```python
from build123d import *

# Parameters (mm, degrees)
SKETCH1_R           = 3.3655
SKETCH1_R_2         = 2.2352
BOSS_EXTRUDE1_DEPTH = 2.54
SKETCH2_R           = 0.6604
SKETCH2_R_2         = 2.31775
SKETCH2_R_3         = 3.3655
SKETCH2_R_4         = 2.2352
SKETCH2_R_5         = 1.143
BOSS_EXTRUDE2_DEPTH = 1.7272
FILLET1_R           = 12.7
SKETCH3_R           = 2.06375
SKETCH3_R_2         = 1.143
CUT_EXTRUDE1_DEPTH  = 1.27
SKETCH8_R           = 0.98
CUT_EXTRUDE4_DEPTH  = 20.062316393


with BuildPart() as part:
    # Sketch1 → Boss-Extrude1 (new body)
    with BuildSketch(Plane(origin=(0, 0, 0), x_dir=(1, 0, 0), z_dir=(0, 1, 0))):
        with Locations(Location((0, 0, 0), (0, 0, 270))):
            Circle(SKETCH1_R)
        with Locations(Location((0, 0, 0), (0, 0, 270))):
            Circle(SKETCH1_R_2, mode=Mode.SUBTRACT)
    extrude(amount=BOSS_EXTRUDE1_DEPTH)

    # Sketch2 → Boss-Extrude2 (add)
    with BuildSketch(Plane(origin=(0, 2.54, 0), x_dir=(1, 0, 0), z_dir=(0, 1, 0))):
        with BuildLine():
            ThreePointArc((-0.713521748, -3.755518873), (-3.8227, 0), (-0.713521748, 3.755518873))
            Line((-0.713521748, 3.755518873), (-16.092265178, 2.307544345))
            ThreePointArc((-16.092265178, 2.307544345), (-14.314807913, 1.713991165), (-13.55725, 0))
            ThreePointArc((-13.55725, 0), (-14.314807913, -1.713991165), (-16.092265178, -2.307544345))
            Line((-16.092265178, -2.307544345), (-0.713521748, -3.755518873))
        make_face()
        with Locations(Location((-12.8778, 0, 0), (0, 0, 270))):
            Circle(SKETCH2_R, mode=Mode.SUBTRACT)
        with Locations(Location((-9.8806, 0, 0), (0, 0, 270))):
            Circle(SKETCH2_R, mode=Mode.SUBTRACT)
        with Locations(Location((-7.1628, 0, 0), (0, 0, 270))):
            Circle(SKETCH2_R, mode=Mode.SUBTRACT)
        with Locations((-15.875, 0)):
            Circle(SKETCH2_R_2)
        with Locations(Location((-15.875, 0, 0), (0, 0, 270))):
            Circle(SKETCH2_R, mode=Mode.SUBTRACT)
        with BuildLine():
            Line((16.092265178, 2.307544345), (0.713521748, 3.755518873))
            ThreePointArc((0.713521748, 3.755518873), (2.944538578, 2.437771083), (3.8227, 0))
            ThreePointArc((3.8227, 0), (2.944538578, -2.437771083), (0.713521748, -3.755518873))
            Line((0.713521748, -3.755518873), (16.092265178, -2.307544345))
            ThreePointArc((16.092265178, -2.307544345), (13.55725, 0), (16.092265178, 2.307544345))
        make_face()
        with Locations(Location((7.1628, 0, 0), (0, 0, 270))):
            Circle(SKETCH2_R, mode=Mode.SUBTRACT)
        with Locations(Location((9.8806, 0, 0), (0, 0, 270))):
            Circle(SKETCH2_R, mode=Mode.SUBTRACT)
        with Locations(Location((12.8778, 0, 0), (0, 0, 270))):
            Circle(SKETCH2_R, mode=Mode.SUBTRACT)
        with Locations((15.875, 0)):
            Circle(SKETCH2_R_2)
        with Locations(Location((15.875, 0, 0), (0, 0, 270))):
            Circle(SKETCH2_R, mode=Mode.SUBTRACT)
        with BuildLine():
            Line((0.713521748, 3.755518873), (0, 3.8227))
            Line((0, 3.8227), (-0.713521748, 3.755518873))
            ThreePointArc((-0.713521748, 3.755518873), (-3.8227, 0), (-0.713521748, -3.755518873))
            Line((-0.713521748, -3.755518873), (0, -3.8227))
            Line((0, -3.8227), (0.713521748, -3.755518873))
            ThreePointArc((0.713521748, -3.755518873), (2.944538578, -2.437771083), (3.8227, 0))
            ThreePointArc((3.8227, 0), (2.944538578, 2.437771083), (0.713521748, 3.755518873))
        make_face()
        with Locations(Location((0, 0, 0), (0, 0, 270))):
            Circle(SKETCH2_R_3, mode=Mode.SUBTRACT)
        with Locations(Location((0, 0, 0), (0, 0, 270))):
            Circle(SKETCH2_R_3)
        with Locations(Location((0, 0, 0), (0, 0, 270))):
            Circle(SKETCH2_R_4, mode=Mode.SUBTRACT)
        with Locations(Location((0, 0, 0), (0, 0, 270))):
            Circle(SKETCH2_R_4)
        with Locations(Location((0, 0, 0), (0, 0, 270))):
            Circle(SKETCH2_R_5, mode=Mode.SUBTRACT)
    extrude(amount=BOSS_EXTRUDE2_DEPTH)

    # Fillet1
    fillet1_edges = [part.edges().sort_by_distance(p)[0] for p in [
        (0, 3.4036, -3.8227),
        (0, 3.4036, 3.8227),
    ]]
    fillet(fillet1_edges, radius=FILLET1_R)

    # Sketch3 → Cut-Extrude1 (cut)
    with BuildSketch(Plane(origin=(0, 4.2672, 0), x_dir=(1, 0, 0), z_dir=(0, 1, 0))):
        with Locations(Location((0, 0, 0), (0, 0, 270))):
            Circle(SKETCH3_R)
        with Locations(Location((0, 0, 0), (0, 0, 270))):
            Circle(SKETCH3_R_2, mode=Mode.SUBTRACT)
    extrude(amount=-CUT_EXTRUDE1_DEPTH, mode=Mode.SUBTRACT)

    # Sketch8 → Cut-Extrude4 (cut, through all)
    with BuildSketch(Plane(origin=(0, 4.2672, 0), x_dir=(1, 0, 0), z_dir=(0, 1, 0))):
        with Locations(Location((10, 0, 0), (0, 0, 270))):
            Circle(SKETCH8_R)
        with Locations(Location((-10, 0, 0), (0, 0, 270))):
            Circle(SKETCH8_R)
    extrude(amount=-CUT_EXTRUDE4_DEPTH, mode=Mode.SUBTRACT)


solid = part.part
```
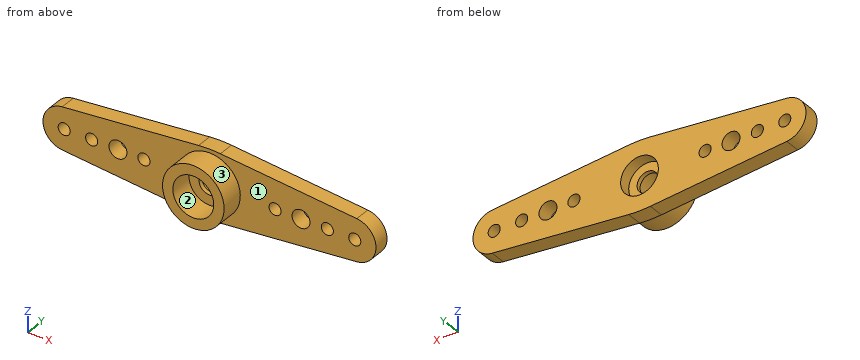
Geometry check sheet. Reference: the model listing, model coordinates, mm. Face numbers are marked on the shaded views. Round coordinates to 2 decimals unless told otherwise and drop trailing zeros. Order: outer loops, then holes, each group sorted by start corner. A loop starts at its lowest first (then second) coordinate and runs counter-clockwise, first axis right, second up. Notation, with made-up numbers: (-32, -38.75) -> (-3, -38.75) arc R14 ccw to (-3, -20.75) -> close; hole circle Ø9 at (-3, 30.25). An arc over 180 degrees is marked (long way). Return JSON: item names as keys, results as strings. Group by question number.
Q1. Section check A-A, the plane x = -10. Record the boundary of the cut face in (y, z).
Q2. Section check C-C, the plane z = 0.25. Count the separate pieces of the cut face and the enclosed holes in it, plus the area to 3 significant figures.
Q3. Section check B-B, the plane y = 1.2. Record the boundary of the cut face in (x, z), plus the area to 3 significant figures.
Q4. Gauge pin test, flat ends, axial feed: pin 1 (2 mm diameter, centred on y = 3, z = 1.5, fed in from -X); pin 2 (2 mm diameter, centred on y = 0.5, z = 3, fed in from +X); pin 3 (1.5 mm diameter, centred on x = 12, y = 2.5, fed in from +Z). Record the tip position at first contact, or that the pin passes through.
Q5. Section check D-D, the plane z = -1.75. Record the boundary of the cut face in (x, y).
Q6. Material ranges on probe 1 along X at (y, z) = (1.8, 0); probe 2 along Y at (x, z) = (3, 3.25); probe 3 along X at (y, z) = (2, -1.5), recorded low to high. Write a range as from..to.
Q7. Release check for a two-part mould opening along Z. For the marked faces 1, 2 and 3 record: released by +Z, released by -Z, zero draft, split by the parting line, or undercut.
Numbers:
{
 "1": {"outline": "(2.54, -2.88) -> (4.27, -2.88) -> (4.27, -0.98) -> (2.54, -0.98) -> close; (2.54, 0.98) -> (4.27, 0.98) -> (4.27, 2.88) -> (2.54, 2.88) -> close"},
 "2": {"separate pieces": "10", "enclosed holes": "0", "area": "43.1 mm^2"},
 "3": {"outline": "circle Ø6.73 at (0, 0); hole circle Ø4.47 at (0, 0)", "area": "19.9 mm^2"},
 "4": {"pin 1": "x = -18.14", "pin 2": "x = 2.71", "pin 3": "z = 2.76"},
 "5": {"outline": "(-17.39, 2.54) -> (-2.87, 2.54) -> (-2.87, 0) -> (-1.39, 0) -> (-1.39, 2.54) -> (1.39, 2.54) -> (1.39, 0) -> (2.87, 0) -> (2.87, 2.54) -> (17.39, 2.54) -> (17.39, 4.27) -> (1.09, 4.27) -> (1.09, 3) -> (-1.09, 3) -> (-1.09, 4.27) -> (-17.39, 4.27) -> close"},
 "6": {"probe 1": "-3.37..-2.24, 2.24..3.37", "probe 2": "2.54..4.27", "probe 3": "-3.01..-1.66, 1.66..3.01"},
 "7": {"face 1": "zero draft", "face 2": "undercut", "face 3": "split by the parting line"}
}
